Autodesk Inventor part; units mm, degrees
ref_plane "YZ Plane" through (0, 0, 0) normal (1, 0, 0) x (0, 1, 0)
ref_plane "XZ Plane" through (0, 0, 0) normal (0, 1, 0) x (-1, 0, 0)
ref_plane "XY Plane" through (0, 0, 0) normal (0, 0, 1) x (1, 0, 0)
sketch "Sketch1" plane through (0, 0, 0) normal (0, 0, 1) x (1, 0, 0)
  line L0 (0, 0) -> (-179.0487, 0)
  line L1 (-179.0487, 0) -> (-179.0487, -1500)
  line L2 (-179.0487, -1500) -> (0, -1500)
  line L3 (0, -1500) -> (0, 0)
  line L4 (-179.0487, -1400) -> (-66, -1400)
  line L5 (-66, -1400) -> (-66, -1395)
  line L6 (-66, -1395) -> (-179.0487, -1395)
  line L7 (-179.0487, -1395) -> (-179.0487, -1400)
  line L8 (-179.0487, -900) -> (-66, -900)
  line L9 (-66, -900) -> (-66, -895)
  line L10 (-66, -895) -> (-179.0487, -895)
  line L11 (-179.0487, -895) -> (-179.0487, -900)
  line L12 (-179.0487, -400) -> (-66, -400)
  line L13 (-66, -400) -> (-66, -395)
  line L14 (-66, -395) -> (-179.0487, -395)
  line L15 (-179.0487, -395) -> (-179.0487, -400)
  circle A0 centre (-179.0487, 0) radius 30
  circle A1 centre (-179.0487, -1500) radius 30
  point P0 (-179.0487, -400)
  point P1 (-149.0487, 0)
  point P2 (-179.0487, -30)
  point P3 (-179.0487, -1470)
  point P4 (-149.0487, -1500)
  dimension "d0" = 1500
  dimension "d1" = 179.0487
  dimension "d2" = 5
  dimension "d4" = 100
  dimension "d7" = 500
  dimension "d23" = 66
  dimension "d24" = 60
extrude "Plate1" add sketch "Sketch1" along normal blind 4 contours L3 L2 A1 L1 L4 L5 L6 L8 L9 L10 L12 L13 L14 A0 L0
sketch "Sketch2" plane through (4, 0, 0) normal (-1, 0, 0) x (0, -1, 0)
  line L0 (1500, 0) -> (0, 0)
  line L1 (0, 0) -> (0, 60)
  line L2 (0, 60) -> (1500, 60)
  line L3 (1500, 60) -> (1500, 0)
edge flange "Flange1" height 60 angle 90 thickness 4 bend radius 4 thickness toward (-1, 0, 0) relief tear relief width 4 relief depth 2 edges at (0, -750, 4) wall of the first edge with corners at (4, -1500, 0) (4, 0, 0) (4, 0, 60) (4, -1500, 60)
bend "Bend1"
corner "Corner1"
chamfer "Corner Chamfer1" distance 3 angle 45 6 edges at (-179.0487, -1400, 2) (-179.0487, -1395, 2) (-179.0487, -900, 2) (-179.0487, -895, 2) (-179.0487, -395, 2) (-179.0487, -400, 2)
equation "\"d1\" = стрингер_глубина_2"
equation "\"d2\" = паз_под_стрингер_толщина"
equation "\"d23\" = паз_под_стрингер_глубина - Thickness"
equation "\"d24\" = 2 * радиус_выреза_под_сварку"
equation "\"d12\" = Thickness"
equation "\"d13\" = BendReliefWidth"
equation "\"d14\" = BendReliefDepth"
equation "\"d15\" = MinimumRemnant"
equation "\"d16\" = TransitionRadius"
equation "\"d17\" = ребро_усилителей"
equation "\"d19\" = BendRadius"
equation "\"d20\" = CornerReliefSize"
equation "\"d21\" = GapSize"
equation "\"d22\" = JacobiRadiusSize"
equation "\"BendRadius\" = Thickness"
equation "\"BendReliefWidth\" = Thickness"
equation "\"BendReliefDepth\" = 0.5 * Thickness"
equation "\"CornerReliefSize\" = 4 * Thickness"
equation "\"MinimumRemnant\" = 2 * Thickness"
equation "\"TransitionRadius\" = BendRadius"
equation "\"JacobiRadiusSize\" = BendRadius"
equation "\"GapSize\" = Thickness"
properties part number "0233 GBK stringer 3" material "Steel"
CAD build for the part. Positions are in the model's coordinates, mm. A direction names the side the tool comes from. Give positions to 0.01 mm unless a question says otherwise; leave off trailing zeros. Order: outer loops, then holes, each group sorted by start corner. A loop starts at its lowest first (then second) coordinate and runs counter-clockwise, first axis right, second up.
(1) Saw through at C-C, the plane z = 33. Give the cut face in (x, y).
(2) Saw through at A-A, the plane x = -116. Give the cut face in (y, z), then the cut area to 3 significant figures.
(3) Tool access for faces 1 (the flat face through (-93, -740, 4)), 2 (the cylindrical face through (-157.604, -20.979, 1.972)): list every direction of +Z, -Z, +X, -X, +Y, -Y with a clear straight run to the whole face (end or side of a thin tool).
(4) Flat gauge pins, fed straight in: pin 1 (2 mm diameter, centred on y = -397.5, z = 2.5, fed in from -X); pin 2 (8 mm diameter, centred on y = -1191.5, z = 12, fed in from -X); pin 3 (10 mm diameter, centred on x = -31.5, y = -514.5, fed in from +Z); pin 4 (8 mm diameter, centred on x = -116, z = 10.5, fed in from +Y). Where does each tip first touch, or does it go through?
(5) Saw through at B-B, the plane y = -1378. Give the cut face in (x, z), then the cut area to 3 significant figures.
(6) Saw through at D-D, the plane x = -23. Give the cut face in (y, z).
(7) Drill centre lines: L1, parallel to Z at x = -22, y = -470; L2, parallel to X at y = -1098.5, z = 7. Where is each one in solid material? Low to high.
Results found:
1. outline: (0, -1500) - (4, -1500) - (4, 0) - (0, 0) - close
2. outline: (-1500, 0) - (-1400, 0) - (-1400, 4) - (-1500, 4) - close; (-1395, 0) - (-900, 0) - (-900, 4) - (-1395, 4) - close; (-895, 0) - (-400, 0) - (-400, 4) - (-895, 4) - close; (-395, 0) - (0, 0) - (0, 4) - (-395, 4) - close
2. area: 5,940 mm2
3. face 1: +Z, -X, +Y, -Y
3. face 2: +Z, -Z, -X, +Y
4. pin 1: stops at x = -66
4. pin 2: stops at x = 0
4. pin 3: stops at z = 4
4. pin 4: passes through
5. outline: (-179.05, 0) - (-4, 0) arc R8 ccw to (4, 8) - (4, 60) - (0, 60) - (0, 8) arc R4 cw to (-4, 4) - (-179.05, 4) - close
5. area: 946 mm2
6. outline: (-1500, 0) - (0, 0) - (0, 4) - (-1500, 4) - close
7. L1: z = 0 to 4
7. L2: x = -0.13 to 3.94
